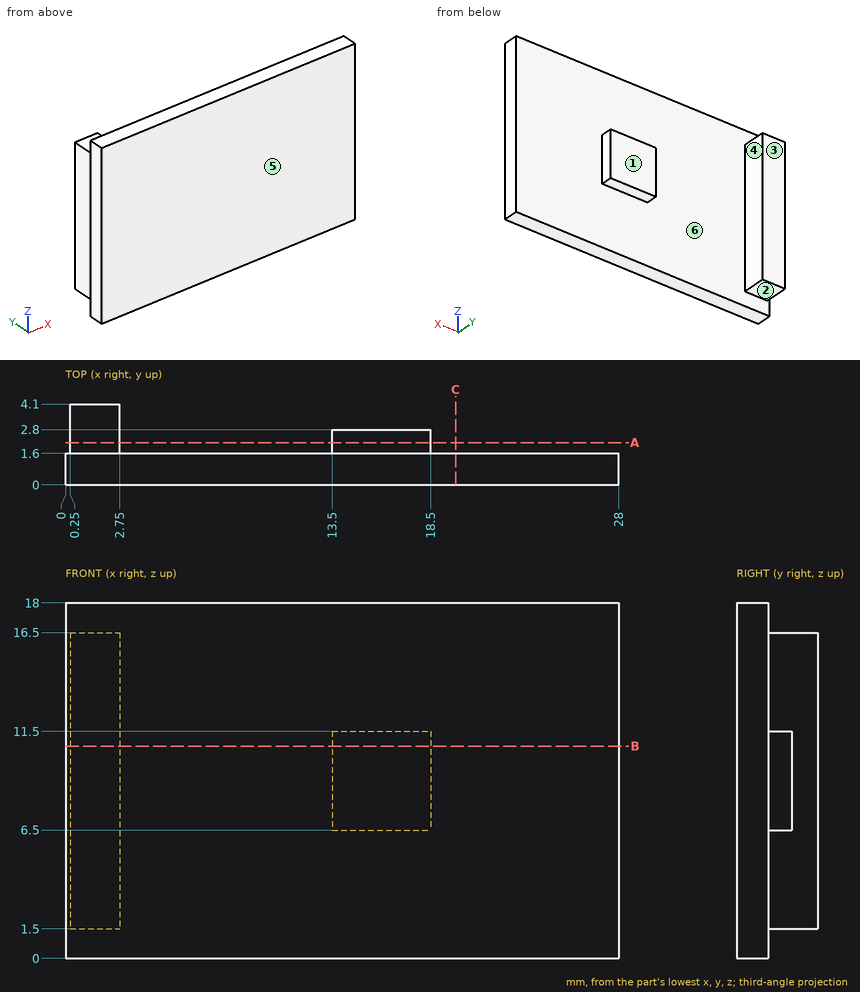
Can you work these out from the drawing? Everything is in mm from the part's minimum corner. A direction names the side the tool comes from. Give positions to 0.01 mm unless a question says otherwise; leave off trailing zeros. Order: outer loops, then holes, each group sorted by start corner. A loop starts at its lowest first (then second) coordinate and runs counter-clockwise, first axis right, second up.
1. Will these pins go through, and if not, where does the flat tip stop? P1, Ø1.2, axis at y = 3, z = 8.5, coming from the +X side; P2, Ø0.7, axis at x = 1.5, y = 2.5, coming from the -Z side; P3, Ø4, axis at x = 9.5, z = 5, coming from the -Y side; P4, Ø1.5, axis at x = 16, z = 9.5, coming from the +Y side.
2. Suppose I cut it at C-C (x = 19.75). List the corners of the cut face in (y, z) for me.
3. For the marked faces 1, 2, 3 and 4, which set-ups out of +Z, -Z, +X, -X, +Y, -Y let a thin tool reach every point of the face, with its end or its side?
4. I need wall thicknesses on L1, parallel to X at y = 1.8, z = 4.5; L2, parallel to Y at x = 19.25, z = 15.75; L3, parallel to Y at x = 15, z = 9.25. Which ranges of each line are inside material? Lowest first, please.
5. Suppose I cut it at B-B (z = 10.75). List the corners of the cut face in (x, y) for me, plus the area to 4 significant figures.
6. We'd pull the mould along X, two halves only. Please class the marked faces 5 and 6: pulls with the +X half, pulls with the -X half, needs draft (parallel to the pull), parting line crosses it, or undercut.
7. Suppose I cut it at A-A (y = 2.15). List the corners of the cut face in (x, z) for me.
Solved:
1. P1: stops at x = 18.5
1. P2: stops at z = 1.5
1. P3: stops at y = 0
1. P4: stops at y = 2.8
2. outline: (0, 0) - (1.6, 0) - (1.6, 18) - (0, 18) - close
3. face 1: +Z, -Z, +X, +Y
3. face 2: -Z, +X, -X, +Y
3. face 3: +Z, -Z, +X, -X, +Y
3. face 4: +Z, -Z, +Y
4. L1: x = 0.25 to 2.75
4. L2: y = 0 to 1.6
4. L3: y = 0 to 2.8
5. outline: (0, 0) - (28, 0) - (28, 1.6) - (18.5, 1.6) - (18.5, 2.8) - (13.5, 2.8) - (13.5, 1.6) - (2.75, 1.6) - (2.75, 4.1) - (0.25, 4.1) - (0.25, 1.6) - (0, 1.6) - close
5. area: 57.05 mm2
6. face 5: needs draft
6. face 6: undercut
7. outline: (0.25, 1.5) - (2.75, 1.5) - (2.75, 16.5) - (0.25, 16.5) - close; (13.5, 6.5) - (18.5, 6.5) - (18.5, 11.5) - (13.5, 11.5) - close
